```python
from build123d import *

# Parameters (mm, degrees)
SKETCH1_W                = 80
SKETCH1_H                = 36
BOSS_EXTRUDE1_DEPTH      = 1.6
SKETCH2_W                = 72
SKETCH2_H                = 24.3
BOSS_EXTRUDE2_DEPTH      = 6.9
SKETCH3_W                = 64
SKETCH3_H                = 13.6
CUT_EXTRUDE1_DEPTH       = 0.5
BOSS_EXTRUDE3_DEPTH      = 4
BOSS_EXTRUDE3_DEPTH_BACK = 7
SKETCH5_W                = 40
SKETCH5_H                = 4
SKETCH7_R                = 1.55
CUT_EXTRUDE2_DEPTH       = 45.418464629
SKETCH8_W                = 40
SKETCH8_H                = 5.4
BOSS_EXTRUDE4_DEPTH      = 10


with BuildPart() as part:
    # Sketch1 → Boss-Extrude1 (new body)
    with BuildSketch(Plane(origin=(0, 0, 0), x_dir=(1, 0, 0), z_dir=(0, 1, 0))):
        Rectangle(SKETCH1_W, SKETCH1_H)
    extrude(amount=BOSS_EXTRUDE1_DEPTH)

    # Sketch2 → Boss-Extrude2 (add)
    with BuildSketch(Plane(origin=(0, 1.6, 0), x_dir=(1, 0, 0), z_dir=(0, 1, 0))):
        with Locations((0, -0.45)):
            Rectangle(SKETCH2_W, SKETCH2_H)
    extrude(amount=BOSS_EXTRUDE2_DEPTH)

    # Sketch3 → Cut-Extrude1 (cut)
    with BuildSketch(Plane(origin=(0, 8.5, 0), x_dir=(1, 0, 0), z_dir=(0, 1, 0))):
        Rectangle(SKETCH3_W, SKETCH3_H)
    extrude(amount=-CUT_EXTRUDE1_DEPTH, mode=Mode.SUBTRACT)

    # Sketch5 → Boss-Extrude3 (add, two sides: drawn at the far end of the back side and taken through both)
    with BuildSketch(Plane(origin=(0, 1.6, 0), x_dir=(1, 0, 0), z_dir=(0, 1, 0)).offset(-BOSS_EXTRUDE3_DEPTH_BACK)):
        with Locations((-13, 16)):
            Rectangle(SKETCH5_W, SKETCH5_H)
    extrude(amount=BOSS_EXTRUDE3_DEPTH + BOSS_EXTRUDE3_DEPTH_BACK)

    # Sketch7 → Cut-Extrude2 (cut, through all)
    with BuildSketch(Plane(origin=(0, 1.6, 0), x_dir=(1, 0, 0), z_dir=(0, 1, 0))):
        with Locations(Location((-37.45, 15.216322293, 0), (0, 0, 270))):
            Circle(SKETCH7_R)
        with Locations(Location((37.45, 15.216322293, 0), (0, 0, 90))):
            Circle(SKETCH7_R)
        with Locations(Location((37.45, -15.216322293, 0), (0, 0, 270))):
            Circle(SKETCH7_R)
        with Locations(Location((-37.45, -15.216322293, 0), (0, 0, 90))):
            Circle(SKETCH7_R)
    extrude(amount=-CUT_EXTRUDE2_DEPTH, mode=Mode.SUBTRACT)

    # Sketch8 → Boss-Extrude4 (add)
    with BuildSketch(Plane.XY.offset(-14)):
        with Locations((-13, -2.7)):
            Rectangle(SKETCH8_W, SKETCH8_H)
    extrude(amount=BOSS_EXTRUDE4_DEPTH)


solid = part.part
```
Geometry: final body of the model. Coordinates: model frame, mm. A direction names the side the tool comes from. Coordinates: 2 decimals unless noted, no trailing zeros. Order: outer loops, then holes, each group sorted by start corner. A loop starts at its lowest first (then second) coordinate and runs counter-clockwise, first axis right, second up.
Item 1: Access query for faces 4 (the face through (-33, -3, -11)), 5 (the face through (-13, 5.6, -16)), 6 (the face through (-33, 4, -16)), 7 (the face through (-1, 5, -11.7)), 8 (the face through (-1, 5, 12.6)). Directions: +Z, -Z, +X, -X, +Y, -Y. A direction counts if a zero-diameter tool reaches every point of the face in a straight line with its end or side. Return the directions, or none.
Answer:
face 4: +Z, -Z, -X, -Y
face 5: -Z, +X, -X, +Y
face 6: -Z, -X, +Y
face 7: +X, -X, +Y
face 8: +Z, +X, -X, +Y
Item 2: Contact query for flat-ended pins moving along their axis: P1, Ø1.5, axis at y = -2.5, z = 11, coming from the -X side; P2, Ø3.5, axis at x = -9.5, y = 6, coming from the +Z side; P3, Ø15, axis at x = -15.5, z = 1.5, coming from the +Y side; P4, Ø0.6, axis at y = 8.5, z = -2.5, coming from the -X side. Output: stop coordinate, or through.
Answer:
P1: passes through
P2: stops at z = 12.6
P3: stops at y = 8.5
P4: stops at x = -36
Item 3: Section query D-D (y = -2.5). Output: boundary loops of the cut face in (x, z), then the cut area to 3 significant figures.
Answer:
outline: (-33, -18) - (7, -18) - (7, -4) - (-33, -4) - close
area: 560 mm2
Item 4: Section query A-A (x = -15). Output: boundary loops of the cut face in (y, z), then the cut area to 3 significant figures.
Answer:
outline: (-5.4, -18) - (5.6, -18) - (5.6, -14) - (1.6, -14) - (1.6, -11.7) - (8.5, -11.7) - (8.5, -6.8) - (8, -6.8) - (8, 6.8) - (8.5, 6.8) - (8.5, 12.6) - (1.6, 12.6) - (1.6, 18) - (0, 18) - (0, -4) - (-5.4, -4) - close
area: 310 mm2
Item 5: Section query C-C (x = 37.45). Output: boundary loops of the cut face in (y, z), then the cut area to 3 significant figures.
Answer:
outline: (0, -18) - (1.6, -18) - (1.6, -16.77) - (0, -16.77) - close; (0, -13.67) - (1.6, -13.67) - (1.6, 13.67) - (0, 13.67) - close; (0, 16.77) - (1.6, 16.77) - (1.6, 18) - (0, 18) - close
area: 47.7 mm2
Item 6: Section query B-B (z = 8). Output: boundary loops of the cut face in (x, y), then the cut area to 3 significant figures.
Answer:
outline: (-40, 0) - (40, 0) - (40, 1.6) - (36, 1.6) - (36, 8.5) - (-36, 8.5) - (-36, 1.6) - (-40, 1.6) - close
area: 625 mm2
Item 7: Material intervals for line 1 along Z through (x, y) = (-21.5, 5.25); line 2 along Y through (x, z) = (-34, -15); line 3 along Y through (x, z) = (26.5, -0.5), sorted ascending.
Answer:
line 1: z = -18 to -14, -11.7 to 12.6
line 2: y = 0 to 1.6
line 3: y = 0 to 8
Item 8: Draft query along X for faces 1 (the face through (-1, 0, 4)), 2 (the face through (7, 4, -16)), 3 (the face through (0, 8, 0)). Return one class per face: released by +X, released by -X, zero draft, split by the parting line, or undercut.
Answer:
face 1: zero draft
face 2: released by +X
face 3: undercut
